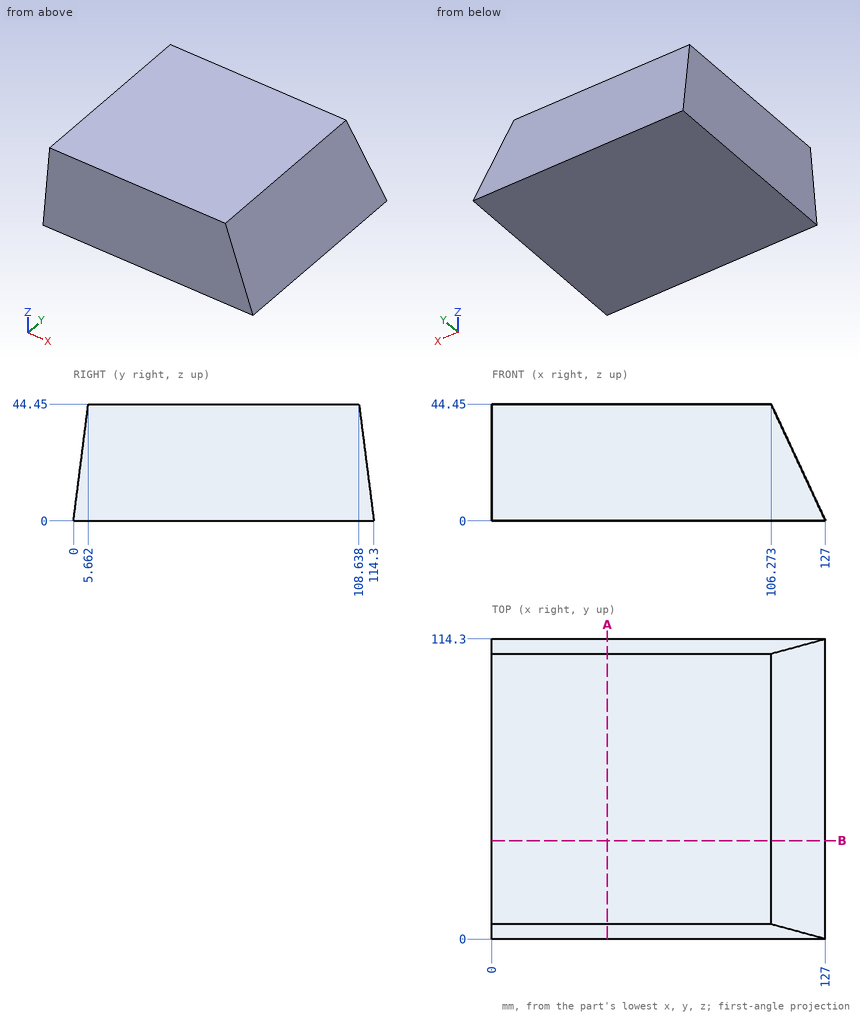
Can you work these out from the drawing? Everything is in mm from the part's minimum corner. Give positions to 0.01 mm unless a question says otherwise; leave off trailing zeros. Order: outer loops, then holes, each group sorted by start corner. A loop starts at its lowest first (then second) coordinate and runs counter-clockwise, first axis right, second up. Notation, with made-up numbers: M 7,72.25 L 42,72.25 A18 cw 42,93.25 Z; hole C 80,1 d3. An arc over 180 degrees is marked long. Write item = value, one per line. Start each with the question number.
Q1. Suppose I cut it at A-A (x = 44). Write out the boundary of the cut face in (y, z), plus the area to 3 significant figures.
Q2. Suppose I cut it at B-B (y = 37.5). Write out the boundary of the cut face in (x, z), plus the area to 3 significant figures.
Q3. I need wall thicknesses on probe 1 along Z at (x, y) = (107.5, 52) (1 decimal); probe 2 along X at (y, z) = (86, 11); probe 3 along Y at (x, z) = (85, 9). Which ranges of each line are inside material? Lowest first, please. Write a range as [from, to].
Q4. Will these pins go through, and if not, where does the flat tip stop? pin 1 Ø5 at (y, z) = (40, 12) entering from +X; pin 2 Ø12 at (y, z) = (75.5, 34.5) entering from +X; pin 3 Ø10 at (x, z) = (111, 6) entering from +Y.
Check result:
q1.outline = M 0,0 L 114.3,0 L 108.64,44.45 L 5.66,44.45 Z
q1.area = 4,830 mm2
q2.outline = M 0,0 L 127,0 L 106.27,44.45 L 0,44.45 Z
q2.area = 5,180 mm2
q3.probe_1 = [0, 41.8]
q3.probe_2 = [0, 121.87]
q3.probe_3 = [1.15, 113.15]
q4.pin_1 = 122.57
q4.pin_2 = 113.71
q4.pin_3 = 114.17
